The drawing under review shows one solid part. Ordinate dimensions are in mm from its lowest x, y, z. A direction names the side the tool comes from. Coordinates: 2 decimals unless noted, no trailing zeros. Write each loop counter-clockwise with the first axis right and the second up, starting at its lowest first coordinate (ties: lowest second). Pieces come first, ordered by that corner, then holes.
Q1. Insertion check: pin 1 (18 mm diameter, centred on x = 25.5, z = 23, fed in from +Y); pin 2 (8 mm diameter, centred on x = 20, y = 16, fed in from -Z); pin 3 (4 mm diameter, centred on x = 14, z = 100, fed in from -Y). Each pin has a flat end and moves straight along its axis. Give the tip position at first contact, or say it passes through.
Q2. Take a section at C-C (x = 8). Give the boundary of the cut face in (y, z), and give its area (3 significant figures).
Q3. Mouldability with a two-part tool opening along Z and no side actions: class the marked faces 3, 4, 5 and 6 as pulls with the +Z half, pulls with the -Z half, needs draft (parallel to the pull), parting line crosses it, or undercut.
Q4. Take a section at A-A (y = 15). State how many separate pieces and enclosed holes the cut face has, and give its area (3 significant figures).
Q5. Take a section at B-B (x = 49.5). Give the boundary of the cut face in (y, z).
Q6. Take a section at D-D (z = 55). Give the boundary of the cut face in (x, y).
Q7. For probe 1 along Y at (x, z) = (57, 121.85); probe 2 along Z at (x, y) = (42.5, 6.25); probe 3 along X at (y, z) = (15, 86.35) (1 decimal), list the stretches that pass through material, from the lowest coordinate up.
Q8. Machinability: for the marked faces 1 and 2, which of the approach directions +Z, -Z, +X, -X, +Y, -Y give a long, thin tool a straight path to every point of the face, cutting with its end or side? Answer none if there is none.
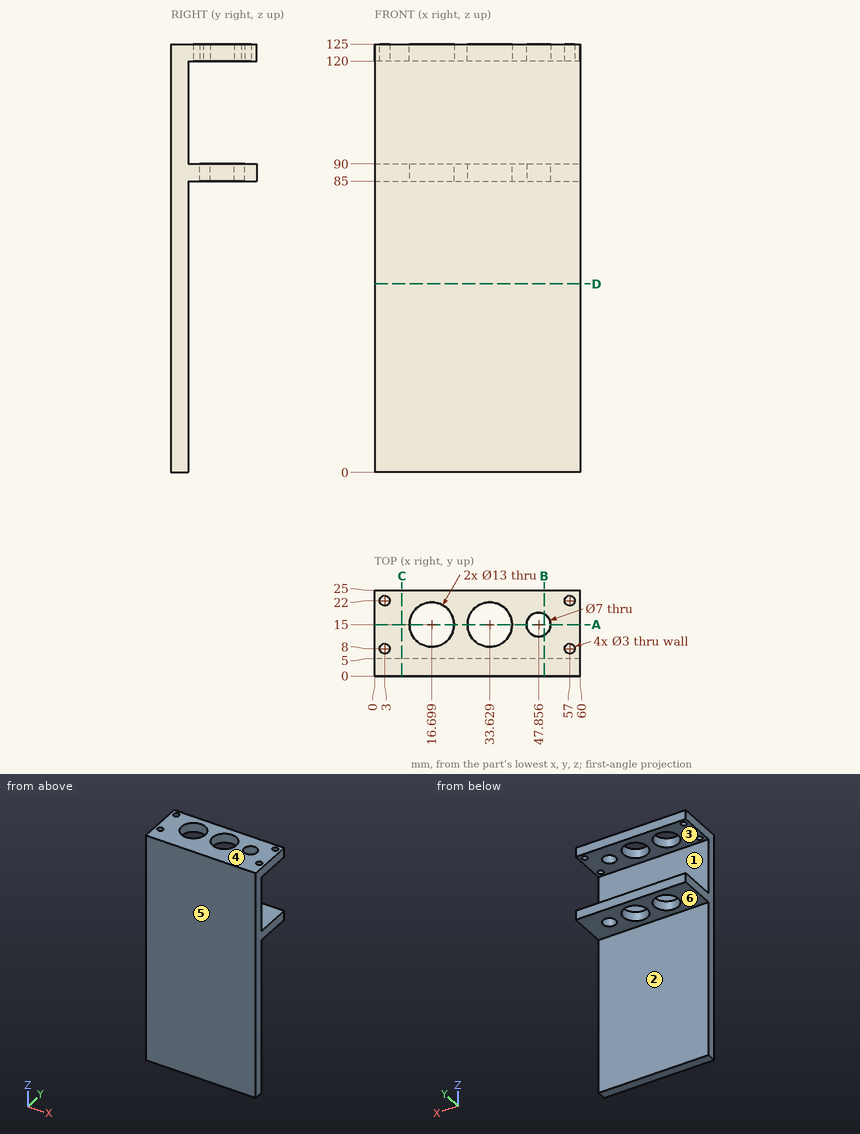
Response:
1. pin 1: stops at y = 5
1. pin 2: stops at z = 85
1. pin 3: stops at y = 0
2. outline: (0, 0) - (5, 0) - (5, 85) - (25, 85) - (25, 90) - (5, 90) - (5, 120) - (25, 120) - (25, 125) - (0, 125) - close
2. area: 825 mm2
3. face 3: undercut
3. face 4: pulls with the +Z half
3. face 5: needs draft
3. face 6: pulls with the -Z half
4. separate pieces: 8
4. enclosed holes: 0
4. area: 270 mm2
5. outline: (0, 0) - (5, 0) - (5, 85) - (11.91, 85) - (11.91, 90) - (5, 90) - (5, 120) - (11.91, 120) - (11.91, 125) - (0, 125) - close; (18.09, 85) - (25, 85) - (25, 90) - (18.09, 90) - close; (18.09, 120) - (25, 120) - (25, 125) - (18.09, 125) - close
6. outline: (0, 0) - (60, 0) - (60, 5) - (0, 5) - close
7. probe 1: y = 0 to 6.5, 9.5 to 20.5, 23.5 to 25
7. probe 2: z = 85 to 90, 120 to 125
7. probe 3: x = 0 to 10.2, 23.2 to 27.1, 40.1 to 44.4, 51.4 to 60
8. face 1: +X, -X, +Y
8. face 2: -Z, +X, -X, +Y
